Source: CAD feature listing. Evaluate the final solid. Frame: model axes, mm. Face numbers are marked on the shaded views. A direction names the side the tool comes from. Coordinates: 2 decimals unless noted, no trailing zeros. Order: outer loops, then holes, each group sorted by start corner. A loop starts at its lowest first (then second) coordinate and runs counter-clockwise, first axis right, second up. Notation, with made-up numbers: (0.25, 63.5) - (25.25, 63.5) arc R14 ccw to (25.25, 84.5) - close; hole circle Ø7 at (63, 25). An arc over 180 degrees is marked (long way). One line per question, with ' | ' between items. Start each with the question number.
(1) Contact query for flat-ended pins moving along their axis: P1, Ø5, axis at x = -13, y = 2.5, coming from the -Z side; P2, Ø4.5, axis at x = -7, y = 0, coming from the +Z side; P3, Ø2.5, axis at x = 2.5, y = -22.5, coming from the -Z side. Output: stop coordinate, or through.
(2) Section B-B (x = 2.5). Return the cut outline in (y, z).
(3) Section C-C (x = -7). Return the cut outline in (y, z).
(4) Access query for the marked faces 1 and 2. Directions: +Z, -Z, +X, -X, +Y, -Y. A direction counts if a zero-diameter tool reaches every point of the face in a straight line with its end or side. Return the directions, or none.
(5) Section A-A (y = -22.5). Return the cut outline in (x, z).
(6) Section D-D (z = -1.75). Return the cut outline in (x, y), then the cut area to 3 significant figures.
(7) Line query: line 1 along Y through (x, z) = (-7, 2.85); line 2 along X through (y, z) = (-18, -1.75); line 3 along Z through (x, y) = (-5, 13). Output: solid intervals per line, ascending.
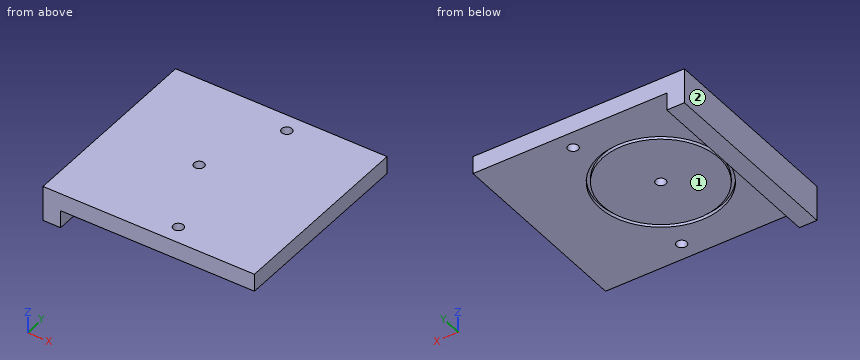
from build123d import *

# Parameters (mm, degrees)
F0_W     = 55
F0_H     = 55
F0_R     = 1.45
F0_R_2   = 17.5
F1_DEPTH = 5
F2_R     = 17.5
F2_R_2   = 16.5
F3_DEPTH = 1
F4_W     = 5
F4_H     = 55
F5_DEPTH = 10


with BuildPart() as f1:
    # F0 (on Top) → F1 (new body)
    with BuildSketch(Plane.XY):
        Rectangle(F0_W, F0_H)
        with Locations((2.5, -22.5)):
            Circle(F0_R, mode=Mode.SUBTRACT)
        with Locations((-7, 0)):
            Circle(F0_R_2, mode=Mode.SUBTRACT)
        with Locations((2.5, 22.5)):
            Circle(F0_R, mode=Mode.SUBTRACT)
        with Locations((-7, 0)):
            Circle(F0_R_2)
        with Locations((-7, 0)):
            Circle(F0_R, mode=Mode.SUBTRACT)
    extrude(amount=F1_DEPTH)

    # F2 (on face) → F3 (cut)
    with BuildSketch(Plane(origin=(0, 0, 0), x_dir=(1, 0, 0), z_dir=(0, 0, -1))):
        with Locations((-7, 0)):
            Circle(F2_R)
        with Locations((-7, 0)):
            Circle(F2_R_2, mode=Mode.SUBTRACT)
    extrude(amount=-F3_DEPTH, mode=Mode.SUBTRACT)

    # F4 (on face) → F5 (join)
    with BuildSketch(Plane.XY.offset(5)):
        with Locations((-30, 0)):
            Rectangle(F4_W, F4_H)
    extrude(amount=-F5_DEPTH)


solid = f1.part
Response values:
1) P1: stops at z = 0 | P2: stops at z = 5 | P3: passes through
2) outline: (-27.5, 0) - (-23.95, 0) - (-23.95, 5) - (-27.5, 5) - close; (-21.05, 0) - (-14.7, 0) - (-14.7, 1) - (-13.49, 1) - (-13.49, 0) - (13.49, 0) - (13.49, 1) - (14.7, 1) - (14.7, 0) - (21.05, 0) - (21.05, 5) - (-21.05, 5) - close; (23.95, 0) - (27.5, 0) - (27.5, 5) - (23.95, 5) - close
3) outline: (-27.5, 0) - (-17.5, 0) - (-17.5, 1) - (-16.5, 1) - (-16.5, 0) - (-1.45, 0) - (-1.45, 5) - (-27.5, 5) - close; (1.45, 0) - (16.5, 0) - (16.5, 1) - (17.5, 1) - (17.5, 0) - (27.5, 0) - (27.5, 5) - (1.45, 5) - close
4) face 1: -Z, +X, +Y, -Y | face 2: +Z, -Z, -X, +Y, -Y
5) outline: (-32.5, -5) - (-27.5, -5) - (-27.5, 0) - (1.05, 0) - (1.05, 5) - (-32.5, 5) - close; (3.95, 0) - (27.5, 0) - (27.5, 5) - (3.95, 5) - close
6) outline: (-32.5, -27.5) - (-27.5, -27.5) - (-27.5, 27.5) - (-32.5, 27.5) - close | area: 275 mm²
7) line 1: y = -27.5 to -1.45, 1.45 to 27.5 | line 2: x = -32.5 to -27.5 | line 3: z = 0 to 5
